Check sheet for the drawn part. Datum: minimum x, y, z corner. Units: mm. A direction names the side the tool comes from. Round coordinates to 2 decimals unless told otherwise and drop trailing zeros. Write each loop counter-clockwise with the first axis right and the second up, starting at its lowest first coordinate (ties: lowest second). Pieces come first, ordered by that corner, then holes.
Item 1: Tool access check on the marked faces 1, 2, 3 and 4. Record the directions out of +Z, -Z, +X, -X, +Y, -Y that give a thin tool (end or side, any length) a straight path to the whole face; none if there is none.
Item 2: Cross-section at D-D on x = 71. Enter the section's corners in (y, z) (1 decimal), plus the area to 3 significant figures.
Item 3: Release check for a two-part mould opening along X. For the marked faces 5, 6 and 7 record: +X half, -X half, draft (parallel to the pull), parting line (faces both ways), or undercut.
Item 4: Cross-section at A-A on z = 29.5. Enter the section's corners in (x, y) (1 decimal), plus the area to 4 significant figures.
Item 5: Go/stop test with flat-tipped pins: pin 1 Ø16.5 at (x, z) = (38.5, 40) entering from -Y; pin 2 Ø10 at (y, z) = (43, 17) entering from +X; pin 3 Ø7 at (y, z) = (4, 7) entering from -X; pin 4 Ø7 at (x, z) = (73, 7) entering from +Y. Record where each tip stops, or that it passes through.
Item 6: Cross-section at C-C on z = 13. Enter the section's corners in (x, y) (1 decimal), plus the area to 3 significant figures.
Item 7: Cross-section at B-B on y = 28. Enter the section's corners in (x, z) (1 decimal), plus the area to 3 significant figures.
Item 8: Material ranges on line 1 (X direction, y = 29.5, z = 43) (1 decimal); line 2 (Y direction, x = 38.5, z = 25.5) (1 decimal); line 3 (Y direction, x = 74.5, z = 22), recorded low to high.
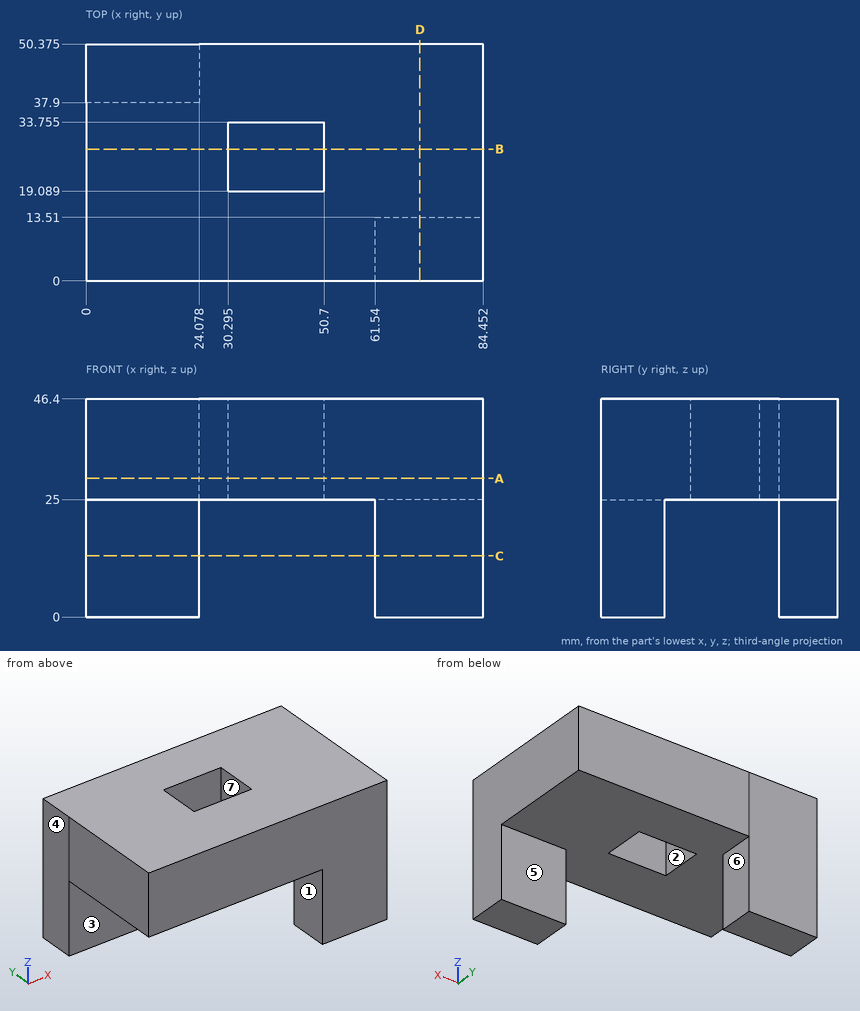
Response values:
1. face 1: -Z, -X, +Y, -Y
1. face 2: +Z, -Z
1. face 3: -Z, +X, -X, -Y
1. face 4: +Z, -Z, -X, +Y, -Y
2. outline: (0, 0) - (13.5, 0) - (13.5, 25) - (50.4, 25) - (50.4, 46.4) - (0, 46.4) - close
2. area: 1,420 mm2
3. face 5: draft
3. face 6: +X half
3. face 7: undercut
4. outline: (0, 0) - (84.5, 0) - (84.5, 50.4) - (0, 50.4) - close; hole (30.3, 19.1) - (50.7, 19.1) - (50.7, 33.8) - (30.3, 33.8) - close
4. area: 3,955 mm2
5. pin 1: stops at y = 0
5. pin 2: stops at x = 24.08
5. pin 3: stops at x = 61.54
5. pin 4: stops at y = 13.51
6. outline: (0, 37.9) - (24.1, 37.9) - (24.1, 50.4) - (0, 50.4) - close; (61.5, 0) - (84.5, 0) - (84.5, 13.5) - (61.5, 13.5) - close
6. area: 610 mm2
7. outline: (0, 25) - (30.3, 25) - (30.3, 46.4) - (0, 46.4) - close; (50.7, 25) - (84.5, 25) - (84.5, 46.4) - (50.7, 46.4) - close
7. area: 1,370 mm2
8. line 1: x = 0 to 30.3, 50.7 to 84.5
8. line 2: y = 0 to 19.1, 33.8 to 50.4
8. line 3: y = 0 to 13.51
